Build history of the part. All positions in model axes, mm. A direction names the side the tool comes from. Round coordinates to 2 decimals unless told otherwise and drop trailing zeros. Write each loop counter-clockwise with the first axis right and the second up, starting at its lowest first coordinate (ties: lowest second). Pieces come first, ordered by that corner, then holes. Notation, with made-up numbers: M -38.5,43 L -10.5,43 A15 ccw -10.5,59 Z; hole C -11,86.25 d3. An arc over 180 degrees is marked long. Write item = value, one per line.
from build123d import *

# Parameters (mm, degrees)
SKETCH_1_W               = 130
SKETCH_1_H               = 10
EXTRUDE_1_DEPTH          = 70
EXTRUDE_1_2_DEPTH        = 70
SKETCH_1_3_W             = 130
SKETCH_1_3_H             = 20
EXTRUDE_2_DEPTH          = 60
SKETCH_3_W               = 20
SKETCH_3_H               = 22.922507492
CUT_EXTRUDE_4_DEPTH      = 130
CUT_EXTRUDE_5_DEPTH      = 153.970585408
CUT_EXTRUDE_5_DEPTH_BACK = 153.970585408
EXTRUDE_3_DEPTH          = 30
SKETCH_1_4_R             = 10
EXTRUDE_4_DEPTH          = 10
SKETCH_1_5_R             = 10
EXTRUDE_5_DEPTH          = 15


with BuildPart() as part:
    # Sketch 1 → Extrude 1 (new body)
    with BuildSketch(Plane(origin=(0, 0, 0), x_dir=(1, 0, 0), z_dir=(0, 1, 0))):
        with Locations((65, -5)):
            Rectangle(SKETCH_1_W, SKETCH_1_H)
    extrude(amount=EXTRUDE_1_DEPTH)



with BuildPart() as body_2:
    # Sketch 1 → Extrude 1 2 (new body)
    with BuildSketch(Plane(origin=(0, 0, 0), x_dir=(1, 0, 0), z_dir=(0, 1, 0))):
        with Locations((65, -35)):
            Rectangle(SKETCH_1_W, SKETCH_1_H)
    extrude(amount=EXTRUDE_1_2_DEPTH)


with BuildPart() as part_1:
    add(part.part)

    add(body_2.part)  # Extrude 2 merges body 2
    # Sketch 1_3 → Extrude 2 (add)
    with BuildSketch(Plane(origin=(0, 0, 0), x_dir=(1, 0, 0), z_dir=(0, 1, 0))):
        with Locations((65, -20)):
            Rectangle(SKETCH_1_3_W, SKETCH_1_3_H)
    extrude(amount=EXTRUDE_2_DEPTH)

    # Sketch 3 → Cut-Extrude 4 (cut)
    with BuildSketch(Plane(origin=(130, 0, 0), x_dir=(0, 0, -1), z_dir=(1, 0, 0))):
        with Locations((-20, 48.538746254)):
            Rectangle(SKETCH_3_W, SKETCH_3_H)
    extrude(amount=-CUT_EXTRUDE_4_DEPTH, mode=Mode.SUBTRACT)

    # Sketch 2 → Cut-Extrude 5 (cut, two sides: drawn at the far end of the back side and taken through both)
    with BuildSketch(Plane.XY.offset(40).offset(-CUT_EXTRUDE_5_DEPTH_BACK)):
        Polygon((130, 70), (0, 70), (130, 47.077492508), align=None)
    extrude(amount=CUT_EXTRUDE_5_DEPTH + CUT_EXTRUDE_5_DEPTH_BACK, mode=Mode.SUBTRACT)

    # Sketch 4 → Extrude 3 (add)
    with BuildSketch(Plane.XY.offset(40)):
        Polygon((130, 37.077492508), (0, 37.077492508), (0, 60), align=None)
    extrude(amount=-EXTRUDE_3_DEPTH)

    # Sketch 1_4 → Extrude 4 (add)
    # profile 1 of 2: a face of its own
    with BuildSketch(Plane(origin=(0, 0, 0), x_dir=(1, 0, 0), z_dir=(0, 1, 0))):
        with BuildLine():
            Line((50, -40), (0, -40))
            Line((0, -40), (0, -60))
            ThreePointArc((0, -60), (7.32233047, -77.67766953), (25, -85))
            Line((25, -85), (75, -85))
            ThreePointArc((75, -85), (57.32233047, -77.67766953), (50, -60))
            Line((50, -60), (50, -40))
        make_face()
        with Locations(Location((25, -60, 0), (0, 0, 270))):
            Circle(SKETCH_1_4_R, mode=Mode.SUBTRACT)
    # profile 2 of 2: a face of its own
    with BuildSketch(Plane(origin=(0, 0, 0), x_dir=(1, 0, 0), z_dir=(0, 1, 0))):
        with BuildLine():
            Line((100, -40), (50, -40))
            Line((50, -40), (50, -60))
            ThreePointArc((50, -60), (57.32233047, -77.67766953), (75, -85))
            ThreePointArc((75, -85), (92.67766953, -77.67766953), (100, -60))
            Line((100, -60), (100, -40))
        make_face()
        with Locations(Location((75, -60, 0), (0, 0, 270))):
            Circle(SKETCH_1_4_R, mode=Mode.SUBTRACT)
    extrude(amount=EXTRUDE_4_DEPTH)

    # Sketch 1_5 → Extrude 5 (add)
    with BuildSketch(Plane(origin=(0, 0, 0), x_dir=(1, 0, 0), z_dir=(0, 1, 0))):
        with BuildLine():
            Line((100, -40), (50, -40))
            Line((50, -40), (50, -60))
            ThreePointArc((50, -60), (57.32233047, -77.67766953), (75, -85))
            ThreePointArc((75, -85), (92.67766953, -77.67766953), (100, -60))
            Line((100, -60), (100, -40))
        make_face()
        with Locations(Location((75, -60, 0), (0, 0, 270))):
            Circle(SKETCH_1_5_R, mode=Mode.SUBTRACT)
    extrude(amount=EXTRUDE_5_DEPTH)


solid = part_1.part
1. Band-saw the part on B-B (z = 31.5). List the corners of the cut face in (x, y), plus the area to 3 significant figures.
Responses:
outline = M 0,0 L 130,0 L 130,47.08 L 0,70 Z
area = 7,610 mm²
2. Flat gauge pins, fed straight in: pin 1 (2 mm diameter, centred on x = 26.5, z = 67.5, fed in from +Y); pin 2 (2 mm diameter, centred on x = 17, z = 66, fed in from +Y); pin 3 (8 mm diameter, centred on x = 84, z = 75, fed in from +Y); pin 4 (4 mm diameter, centred on x = 61.5, z = 29, fed in from +Y). Where does each tip first touch, or does it go through?
Responses:
pin_1 = through
pin_2 = 10
pin_3 = 15
pin_4 = 59.46
3. Band-saw the part on A-A (y = 62.5). List the corners of the cut face in (x, z), plus the area to 3 significant figures.
Responses:
outline = M 0,0 L 42.53,0 L 42.53,10 L 0,10 Z; M 0,30 L 42.53,30 L 42.53,40 L 0,40 Z
area = 851 mm²
4. Mould opens along Z. For faces 1 (the face through (130, 23, 20)), 2 (the face through (25, 5, 50)), 3 (the face through (83.032, 9.062, 83.675)) say: pulls with the +Z half, pulls with the -Z half, needs draft (parallel to the pull), parting line crosses it, or undercut.
Responses:
face_1 = needs draft
face_2 = undercut
face_3 = pulls with the +Z half
5. Tool access for faces 4 (the face through (64, 15, 62)), 5 (the face through (37, 10, 62)), 6 (the face through (64.09, 58.7, 34.93)), 7 (the face through (0, 35, 23)), 8 (the face through (65, 51, 30)): list every direction of +Z, -Z, +X, -X, +Y, -Y with a clear straight run to the whole face (end or side of a thin tool).
Responses:
face_4 = +Z, +X, -X, +Y
face_5 = +Z, -X, +Y
face_6 = +Z, -Z, +X, +Y
face_7 = +Z, -Z, -X, +Y, -Y
face_8 = +X, +Y
6. Probe probe 1 along X at (y, z) = (8, 60); probe 2 along Y at (x, z) = (50, 69.5); probe 3 along Z at (x, y) = (69, 35). List the from-to ranges inside material, lowest first.
Responses:
probe_1 = 0 to 15, 35 to 65, 85 to 100
probe_2 = 0 to 10
probe_3 = 0 to 40
7. Band-saw the part on C-C (x = 48). List the corners of the cut face in (y, z).
Responses:
outline = M 0,0 L 61.54,0 L 61.54,10 L 51.54,10 L 51.54,30 L 61.54,30 L 61.54,40 L 10,40 L 10,85 L 0,85 Z
8. Band-saw the part on D-D (y = 50.5). List the corners of the cut face in (x, z), plus the area to 3 significant figures.
Responses:
outline = M 0,0 L 110.59,0 L 110.59,10 L 53.88,10 L 53.88,30 L 110.59,30 L 110.59,40 L 0,40 Z
area = 3,290 mm²
